from build123d import *

# Parameters (mm, degrees)
F0_W     = 400
F0_H     = 60
F1_DEPTH = 25
F2_R     = 29.99999
F4_DEPTH = 25


# Not quite as in the source:
# - a fillet or chamfer is up to 0.001 mm smaller than in the source, because OpenCascade refuses the exact size


with BuildPart() as f1:
    # F0 (on Front) → F1 (new body)
    with BuildSketch(Plane.XZ):
        Rectangle(F0_W, F0_H)
    extrude(amount=F1_DEPTH)

    # F2 (radius 30 in the source; OpenCascade refuses exactly that, so slightly less here)
    f2_edges = [f1.edges().sort_by_distance(p)[0] for p in [
        (-200, -12.5, 30),
        (-200, -12.5, -30),
        (200, -12.5, 30),
        (200, -12.5, -30),
    ]]
    fillet(f2_edges, radius=F2_R)

    # F3 (on face) → F4 (cut)
    with BuildSketch(Plane.XZ.offset(25)):
        with BuildLine():
            ThreePointArc((150, 0), (170, -20), (190, 0))
            ThreePointArc((190, 0), (170, 20), (150, 0))
        make_face()
    extrude(amount=-F4_DEPTH, mode=Mode.SUBTRACT)


solid = f1.part
Input: part model. Units: mm. Frame: model coordinates. Coordinates: 2 decimals unless noted, no trailing zeros. Order: outer loops, then holes, each group sorted by start corner. A loop starts at its lowest first (then second) coordinate and runs counter-clockwise, first axis right, second up.
1. Cut plane C-C, the plane z = 26. Return loops of the section in (x, y), plus the area to 3 significant figures.
Checked values:
outline: (-184.97, -25) - (184.97, -25) - (184.97, 0) - (-184.97, 0) - close
area: 9,250 mm2
2. Draft query along X for faces 1 (the cylindrical face through (150.02, -12.68, 0.88)), 2 (the flat face through (-2, -12, -30)), 3 (the cylindrical face through (-191.445, -12.675, 20.979)). Return one class per face: +X half, -X half, draft (parallel to the pull), parting line (faces both ways), or undercut.
Checked values:
face 1: undercut
face 2: draft
face 3: -X half
3. Cut plane B-B, the plane z = -4. Return loops of the section in (x, y), plus the area to 3 significant figures.
Checked values:
outline: (-199.73, -25) - (150.4, -25) - (150.4, 0) - (-199.73, 0) - close; (189.6, -25) - (199.73, -25) - (199.73, 0) - (189.6, 0) - close
area: 9,010 mm2
4. Ray query, line 1 along X through (y, z) = (-22, -14); line 2 along X through (y, z) = (-23, 8); line 3 along Z through (x, y) = (179.5, -19.25). Return the intervals inside material, ascending.
Checked values:
line 1: x = -196.53 to 155.72, 184.28 to 196.53
line 2: x = -198.91 to 151.67, 188.33 to 198.91
line 3: z = -28.46 to -17.6, 17.6 to 28.46
